Geometry: final body of the model. Coordinates: model frame, mm. Give positions to 0.01 mm unless a question says otherwise; leave off trailing zeros. Write each loop counter-clockwise with the first axis right and the second up, starting at its lowest first coordinate (ties: lowest second). Pieces come first, ordered by that corner, then holes. Notation, with made-up numbers: (29.5, -7.5) -> (58.5, -7.5) arc R14 cw to (58.5, 7.5) -> close; hole circle Ø8 at (82.25, 26). An arc over 180 degrees is marked (long way). Answer in a Markdown table with one row per item. Add a question column.
from build123d import *

# Parameters (mm, degrees)
BOSS_EXTRUDE1_DEPTH     = 1.6
FILLET1_R               = 1
BOSS_EXTRUDE2_DEPTH     = 1.6
CUT_EXTRUDE1_DEPTH      = 282.031243815
CUT_EXTRUDE1_DEPTH_BACK = 282.031243815
SKETCH2_W               = 12.4
SKETCH2_H               = 5.75
SKETCH2_W_2             = 3.98
SKETCH2_H_2             = 1.7


with BuildPart() as part:
    # Sketch1 → Boss-Extrude1 (new body)
    with BuildSketch(Plane.XY):
        with BuildLine():
            Line((21.213203436, 24), (0, 2.786796564))
            Line((0, 2.786796564), (0, 0))
            Line((0, 0), (42, 0))
            Line((42, 0), (42, 11))
            ThreePointArc((42, 11), (43.171572875, 13.828427125), (46, 15))
            Line((46, 15), (234, 15))
            ThreePointArc((234, 15), (236.828427125, 13.828427125), (238, 11))
            Line((238, 11), (238, 0))
            Line((238, 0), (280, 0))
            Line((280, 0), (280, 2.786796564))
            Line((280, 2.786796564), (258.786796564, 24))
            Line((258.786796564, 24), (21.213203436, 24))
        make_face()
    extrude(amount=BOSS_EXTRUDE1_DEPTH)

    # Fillet1
    fillet1_edges = [part.edges().sort_by_distance(p)[0] for p in [
        (0, 0, 0.8),
        (0, 2.786796564, 0.8),
        (21.213203436, 24, 0.8),
        (258.786796564, 24, 0.8),
        (280, 2.786796564, 0.8),
        (280, 0, 0.8),
    ]]
    fillet(fillet1_edges, radius=FILLET1_R)

    # Sketch1<3> → Boss-Extrude2 (add)
    with BuildSketch(Plane.XY):
        with BuildLine():
            Line((42, 11), (42, 0))
            Line((42, 0), (238, 0))
            Line((238, 0), (238, 11))
            ThreePointArc((238, 11), (236.828427125, 13.828427125), (234, 15))
            Line((234, 15), (46, 15))
            ThreePointArc((46, 15), (43.171572875, 13.828427125), (42, 11))
        make_face()
    extrude(amount=BOSS_EXTRUDE2_DEPTH)

    # Sketch2 → Cut-Extrude1 (cut, two sides: drawn at the far end of the back side and taken through both)
    with BuildSketch(Plane.XY.offset(-CUT_EXTRUDE1_DEPTH_BACK)):
        with Locations((52.2, 9.675)):
            Rectangle(SKETCH2_W, SKETCH2_H)
        with Locations((70, 7.65)):
            Rectangle(SKETCH2_W_2, SKETCH2_H_2)
        with Locations((90, 7.65)):
            Rectangle(SKETCH2_W_2, SKETCH2_H_2)
        with Locations((110, 7.65)):
            Rectangle(SKETCH2_W_2, SKETCH2_H_2)
        with Locations((150, 7.65)):
            Rectangle(SKETCH2_W_2, SKETCH2_H_2)
        with Locations((170, 7.65)):
            Rectangle(SKETCH2_W_2, SKETCH2_H_2)
        with Locations((190, 7.65)):
            Rectangle(SKETCH2_W_2, SKETCH2_H_2)
        with Locations((210, 7.65)):
            Rectangle(SKETCH2_W_2, SKETCH2_H_2)
        with Locations((227.8, 9.675)):
            Rectangle(SKETCH2_W, SKETCH2_H)
        with Locations((130, 7.65)):
            Rectangle(SKETCH2_W_2, SKETCH2_H_2)
    extrude(amount=CUT_EXTRUDE1_DEPTH + CUT_EXTRUDE1_DEPTH_BACK, mode=Mode.SUBTRACT)


solid = part.part
Q1. Pull-direction query (Z, two-part tool) for faces 1 (the flat face through (269.538, 13.249, 0.789)), 2 (the flat face through (138, 12, 1.6)), 3 (the flat face through (138, 12, 0)); classes: +Z half, -Z half, draft (parallel to the pull), parting line (faces both ways), or undercut.
Q2. Section A-A on z = 1.25. Count the separate pieces of the cut face and the enclosed holes in it, and give its area (3 significant figures).
Q3. Line query: probe 1 along Y at (x, z) = (110.5, 0.3); probe 2 along X at (y, z) = (12.5, 0.25); probe 3 along X at (y, z) = (11.25, 1.5). Output: solid intervals per line, ascending. Write a range as from..to.
Q4. Section B-B on y = 20.5. Return loops of the section in (x, z).
Q5. Contact query for flat-ended pins moving along their axis: pin 1 Ø0.5 at (y, z) = (8, 1) entering from +X; pin 2 Ø0.8 at (y, z) = (7.5, 1) entering from +X; pin 3 Ø0.8 at (y, z) = (8.5, 1) entering from +X. Output: stop coordinate, or through.
Checks:
| question | item | result |
|---|---|---|
| 1 | face 1 | draft |
| 1 | face 2 | +Z half |
| 1 | face 3 | -Z half |
| 2 | separate pieces | 1 |
| 2 | enclosed holes | 10 |
| 2 | area | 6,070 mm^2 |
| 3 | probe 1 | 0..6.8, 8.5..24 |
| 3 | probe 2 | 9.71..46, 58.4..221.6, 234..270.29 |
| 3 | probe 3 | 8.46..46, 58.4..221.6, 234..271.54 |
| 4 | outline | (17.71, 0) -> (262.29, 0) -> (262.29, 1.6) -> (17.71, 1.6) -> close |
| 5 | pin 1 | x = 275.04 |
| 5 | pin 2 | x = 275.69 |
| 5 | pin 3 | x = 274.69 |
